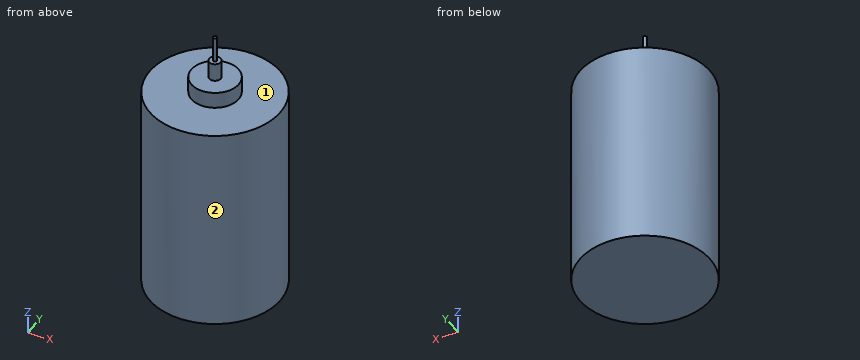
```python
from build123d import *

# Parameters (mm, degrees)
SKETCH1_R           = 17.9
BOSS_EXTRUDE1_DEPTH = 57
SKETCH2_R           = 6.5
BOSS_EXTRUDE2_DEPTH = 4.5
SKETCH3_R           = 1.5875
BOSS_EXTRUDE3_DEPTH = 12
CUT_EXTRUDE1_START  = -7
SKETCH4_R           = 1.5875
SKETCH4_R_2         = 0.518930275
CUT_EXTRUDE1_DEPTH  = 7


with BuildPart() as part:
    # Sketch1 → Boss-Extrude1 (new body)
    with BuildSketch(Plane.XY):
        with Locations(Location((0, 0, 0), (0, 0, 180))):
            Circle(SKETCH1_R)
    extrude(amount=BOSS_EXTRUDE1_DEPTH)

    # Sketch2 → Boss-Extrude2 (add)
    with BuildSketch(Plane.XY.offset(57)):
        Circle(SKETCH2_R)
    extrude(amount=BOSS_EXTRUDE2_DEPTH)

    # Sketch3 → Boss-Extrude3 (add)
    with BuildSketch(Plane.XY.offset(61.5)):
        Circle(SKETCH3_R)
    extrude(amount=BOSS_EXTRUDE3_DEPTH)

    # Sketch4 → Cut-Extrude1 (cut)
    with BuildSketch(Plane.XY.offset(73.5).offset(CUT_EXTRUDE1_START)):
        Circle(SKETCH4_R)
        Circle(SKETCH4_R_2, mode=Mode.SUBTRACT)
    extrude(amount=CUT_EXTRUDE1_DEPTH, mode=Mode.SUBTRACT)


solid = part.part
```
Here's how the part is built. I have some questions about the finished solid (model axes, mm). Face numbers are marked on the shaded views. A direction names the side the tool comes from. Round coordinates to 2 decimals unless told otherwise and drop trailing zeros. Loops run counter-clockwise (first coordinate to the right, second up) from the corner with the lowest first, then second, coordinate; pieces in that order, holes last. Notation, with made-up numbers: (16, -27) -> (29, -27) arc R31 ccw to (29, 9) -> close; hole circle Ø8 at (24, 32). An arc over 180 degrees is marked (long way). Answer as CSV lines item,"result".
1. If we section it at A-A on x = 4: Please give me the cut outline in (y, z), plus the area to 3 significant figures.
Final values:
outline,"(-17.45, 0) -> (17.45, 0) -> (17.45, 57) -> (5.12, 57) -> (5.12, 61.5) -> (-5.12, 61.5) -> (-5.12, 57) -> (-17.45, 57) -> close"
area,"2,040 mm^2"
2. For pin 1 (12 mm diameter, centred on x = -13, y = -0.5, fed in from -Z); pin 2 (2 mm diameter, centred on x = -1.5, z = 43, fed in from +Y); pin 3 (8 mm diameter, centred on y = -5, z = 50.5, fed in from +X); pin 4 (10 mm diameter, centred on y = 13, z = 45.5, fed in from +X), each with a flat end and sliding along its axis, tell me the tip position at first contact or that it passes through.
Final values:
pin 1,"stops at z = 0"
pin 2,"stops at y = 17.89"
pin 3,"stops at x = 17.87"
pin 4,"stops at x = 16.01"
3. If I drill on L1, parallel to Z at x = 10.5, y = -4; L2, parallel to X at y = 10.5, z = 36; L3, parallel to Y at x = -16, z = 5, over which ranges is the centre line in solid material (lowest first)?
Final values:
L1,"z = 0 to 57"
L2,"x = -14.5 to 14.5"
L3,"y = -8.03 to 8.03"
4. If we section it at B-B on z = 36.5: Please give me the cut outline in (x, y), plus the area to 3 significant figures.
Final values:
outline,"circle Ø35.8 at (0, 0)"
area,"1,010 mm^2"
5. If we section it at D-D on x = -9: Please give me the cut outline in (y, z).
Final values:
outline,"(-15.47, 0) -> (15.47, 0) -> (15.47, 57) -> (-15.47, 57) -> close"
6. If we section it at C-C on y = 15.5: Please give me the cut outline in (x, z), plus the area to 3 significant figures.
Final values:
outline,"(-8.95, 0) -> (8.95, 0) -> (8.95, 57) -> (-8.95, 57) -> close"
area,"1,020 mm^2"
7. Which directions (+Z, -Z, +X, -X, +Y, -Y) give clear straight access to the entire face, cutting with the end or side of a thin tool? Please do the marked faces 1 and 2.
Final values:
face 1,"+Z"
face 2,"+Z, -Z"
